Read the model definition and answer for the solid it produces. Units are mm, in the model's axes. Face numbers are marked on the shaded views. A direction names the side the tool comes from. Coordinates: 2 decimals unless noted, no trailing zeros. Loops run counter-clockwise (first coordinate to the right, second up) from the corner with the lowest first, then second, coordinate; pieces in that order, holes last. Notation, with made-up numbers: (62.25, 50) -> (110.25, 50) arc R13 ccw to (110.25, 74) -> close; hole circle Ø5 at (-17, 49). An arc over 180 degrees is marked (long way). Answer as CSV lines item,"result".
Autodesk Inventor part; units mm, degrees
ref_plane "YZ Plane" through (0, 0, 0) normal (1, 0, 0) x (0, 1, 0)
ref_plane "XZ Plane" through (0, 0, 0) normal (0, 1, 0) x (-1, 0, 0)
ref_plane "XY Plane" through (0, 0, 0) normal (0, 0, 1) x (1, 0, 0)
sketch "Arduino Uno" plane through (0, 0, 0) normal (0, 0, 1) x (1, 0, 0)
  line L0 (0, 0) -> (68.6, 0)
  line L1 (68.6, 0) -> (68.6, 53.3)
  line L2 (68.6, 53.3) -> (0, 53.3)
  line L3 (0, 53.3) -> (0, 0)
  circle A0 centre (14, 2.5) radius 1.6
  circle A1 centre (15.3, 50.7) radius 1.6
  circle A2 centre (66.1, 5.1) radius 1.6
  circle A3 centre (66.1, 33) radius 1.6
  dimension "d6" = 68.6
  dimension "d7" = 53.3
  dimension "d8" = 3.2
  dimension "d12" = 14
  dimension "d13" = 2.5
  dimension "d14" = 3.2
  dimension "d15" = 1.3
  dimension "d16" = 3.2
  dimension "d18" = 2.5
  dimension "d19" = 5.1
  dimension "d20" = 3.2
  dimension "d21" = 27.9
  dimension "d22" = 2.5
  dimension "d26" = 2.6
sketch "Sketch2" plane through (0, 0, 0) normal (0, 0, 1) x (1, 0, 0)
  line L0 (-7.6136, -10.2044) -> (-7.6136, 63.0956)
  line L1 (-7.6136, 63.0956) -> (106.3864, 63.0956)
  line L2 (106.3864, 63.0956) -> (106.3864, -10.2044)
  line L3 (106.3864, -10.2044) -> (-7.6136, -10.2044)
  dimension "d29" = 114
  dimension "d39" = 73.3
extrude "Back Plate" add sketch "Sketch2" against normal blind 10
extrude "Uno Mounting Holes" cut sketch "Arduino Uno" against normal blind 5 contours A0 | A1 | A2 | A3
sketch "3.5\" TFT LCD Screen" plane through (0, 0, 0) normal (0, 0, 1) x (1, 0, 0)
  line L0 (88.6005, 0.0003) -> (88.6005, 53.3003)
  line L1 (88.6005, 53.3003) -> (10.6005, 53.3003)
  line L2 (10.6005, 53.3003) -> (10.6005, 0.0003)
  line L3 (10.6005, 0.0003) -> (88.6005, 0.0003)
  circle A0 centre (66.1, 5.1) radius 1.6
  circle A1 centre (14, 2.5) radius 1.6
  circle A2 centre (15.3, 50.7) radius 1.6
  circle A3 centre (66.1, 33) radius 1.6
  line L4 (-7.6136, -10.2044) -> (-7.6136, 63.0956)
  line L5 (106.3864, -10.2044) -> (-7.6136, -10.2044)
  line L6 (106.3864, 63.0956) -> (106.3864, -10.2044)
  line L7 (-7.6136, 63.0956) -> (106.3864, 63.0956)
  point P0 (0, 0)
  point P1 (68.6, 0)
  dimension "d35" = 78
  dimension "d36" = 53.3
  dimension "d37" = 78
  dimension "d38" = 53.3
sketch "SD Card Slot" plane through (0, 0, 0) normal (0, 0, 1) x (1, 0, 0)
  line L0 (43.3864, 9.1) -> (-7.6136, 9.1)
  line L1 (-7.6136, 9.1) -> (-7.6136, 44.1)
  line L2 (-7.6136, 44.1) -> (43.3864, 44.1)
  line L3 (43.3864, 44.1) -> (43.3864, 9.1)
  circle A0 centre (14, 2.5) radius 1.6
  line L4 (-7.6136, -10.2044) -> (-7.6136, 63.0956)
  circle A1 centre (15.3, 50.7) radius 1.6
  point P0 (0, 0)
  dimension "d41" = 35
  dimension "d42" = 51
  dimension "d44" = 6.6
  dimension "d45" = 0
sketch "Sketch5" plane through (0, 0, 0) normal (0, 0, 1) x (1, 0, 0)
  line L0 (43.3864, 9.1) -> (-7.6136, 9.1)
  line L1 (43.3864, 44.1) -> (43.3864, 9.1)
  line L2 (-7.6136, 44.1) -> (43.3864, 44.1)
  line L3 (-7.6136, 9.1) -> (-7.6136, 44.1)
  line L4 (44.3864, 8.1) -> (44.3864, 45.1)
  line L5 (44.3864, 8.1) -> (-7.6136, 8.1)
  line L6 (-7.6136, -10.2044) -> (-7.6136, 63.0956)
  line L7 (44.3864, 45.1) -> (-7.6136, 45.1)
  line L8 (-7.6136, 45.1) -> (-7.6136, 47.6)
  line L9 (-7.6136, 47.6) -> (47.3864, 47.6)
  line L10 (-7.6136, 8.1) -> (-7.6136, 5.6)
  line L11 (-7.6136, 5.6) -> (47.3864, 5.6)
  line L12 (47.3864, 5.6) -> (47.3864, 47.6)
  point P0 (0, 0)
  dimension "d47" = 2.5
  dimension "d48" = 55
  dimension "d49" = 2.5
extrude "SD Card Slot Slot" add sketch "Sketch5" along normal blind 10 contours L5 L4 L7 L6 L9 L12 L11
sketch "Sketch6" plane through (47.3864, 5.6, 0) normal (1, 0, 0) x (0, 0, -1)
  line L0 (0, 42) -> (0, 0)
  line L1 (0, 42) -> (-10, 42)
  line L2 (-10, 0) -> (-10, 42)
  line L3 (0, 0) -> (-10, 0)
  line L4 (-6, 38) -> (-4, 38)
  line L5 (-4, 38) -> (-4, 4)
  line L6 (-4, 4) -> (-6, 4)
  line L7 (-6, 4) -> (-6, 38)
  point P0 (0, -5.6)
  dimension "d52" = 4
extrude "SD Ribbon Slot" cut sketch "Sketch6" against normal through all contours L4 L5 L6 L7
fillet "1.2mm Fillet" radius 1.2 7 edges at (19.8864, 47.6, 0) (19.8864, 5.6, 0) (47.3864, 26.6, 0) (47.3864, 5.6, 5) (47.3864, 47.6, 5) (44.3864, 45.1, 5) (44.3864, 8.1, 5)
sketch "Sketch7" plane through (0, 0, 0) normal (0, 0, 1) x (1, 0, 0)
  line L0 (106.3864, -10.2044) -> (101.3864, -10.2044)
  line L1 (101.3864, -10.2044) -> (101.3864, -5.2044)
  line L2 (101.3864, -5.2044) -> (106.3864, -5.2044)
  line L3 (106.3864, -5.2044) -> (106.3864, -10.2044)
  line L4 (49.3864, -10.2044) -> (49.3864, 80.0118)
  line L5 (-7.6136, 63.0956) -> (106.3864, 63.0956)
  line L6 (106.3864, 26.4456) -> (-34.6963, 26.4456)
  line L7 (-7.6136, -10.2044) -> (-2.6136, -10.2044)
  line L8 (-2.6136, -10.2044) -> (-2.6136, -5.2044)
  line L9 (-2.6136, -5.2044) -> (-7.6136, -5.2044)
  line L10 (-7.6136, -5.2044) -> (-7.6136, -10.2044)
  line L11 (106.3864, 63.0956) -> (101.3864, 63.0956)
  line L12 (101.3864, 63.0956) -> (101.3864, 58.0956)
  line L13 (101.3864, 58.0956) -> (106.3864, 58.0956)
  line L14 (106.3864, 58.0956) -> (106.3864, 63.0956)
  line L15 (-7.6136, 63.0956) -> (-2.6136, 63.0956)
  line L16 (-2.6136, 63.0956) -> (-2.6136, 58.0956)
  line L17 (-2.6136, 58.0956) -> (-7.6136, 58.0956)
  line L18 (-7.6136, 58.0956) -> (-7.6136, 63.0956)
  point P0 (0, 0)
  point P1 (0, 52.8913)
  dimension "d56" = 5
  dimension "d57" = 5
  dimension "d58" = 57
  dimension "d59" = 36.65
extrude "Pillars" add sketch "Sketch7" along normal blind 31
sketch "Sketch8" plane through (0, 0, 31) normal (0, 0, 1) x (1, 0, 0)
  line L0 (101.3864, -10.2044) -> (-2.6136, -10.2044)
  line L1 (-7.6136, -5.2044) -> (-2.6136, -5.2044)
  line L2 (101.3864, -10.2044) -> (-2.6136, -10.2044)
  line L3 (-2.6136, -10.2044) -> (-2.6136, -5.2044)
  line L4 (-2.6136, -5.2044) -> (101.3864, -5.2044)
  line L5 (101.3864, -5.2044) -> (101.3864, -10.2044)
  line L6 (101.3864, 63.0956) -> (101.3864, 58.0956)
  line L7 (106.3864, 63.0956) -> (106.3864, -10.2044)
  line L8 (101.3864, 58.0956) -> (106.3864, 58.0956)
  line L9 (106.3864, 58.0956) -> (106.3864, -5.2044)
  line L10 (106.3864, -5.2044) -> (101.3864, -5.2044)
  line L11 (101.3864, -5.2044) -> (101.3864, 58.0956)
  line L12 (-7.6136, 58.0956) -> (-2.6136, 58.0956)
  line L13 (-7.6136, 63.0956) -> (106.3864, 63.0956)
  line L14 (-2.6136, 58.0956) -> (101.3864, 58.0956)
  line L15 (101.3864, 58.0956) -> (101.3864, 63.0956)
  line L16 (101.3864, 63.0956) -> (-2.6136, 63.0956)
  line L17 (-2.6136, 63.0956) -> (-2.6136, 58.0956)
  line L18 (-2.6136, 58.0956) -> (-7.6136, 58.0956)
  line L19 (-7.6136, 58.0956) -> (-7.6136, -5.2044)
  line L20 (-7.6136, -5.2044) -> (-2.6136, -5.2044)
  line L21 (-2.6136, -5.2044) -> (-2.6136, 58.0956)
  point P0 (0, 0)
extrude "Beams (Will they print?)" [suppressed]
properties part number "Back Plate test03"
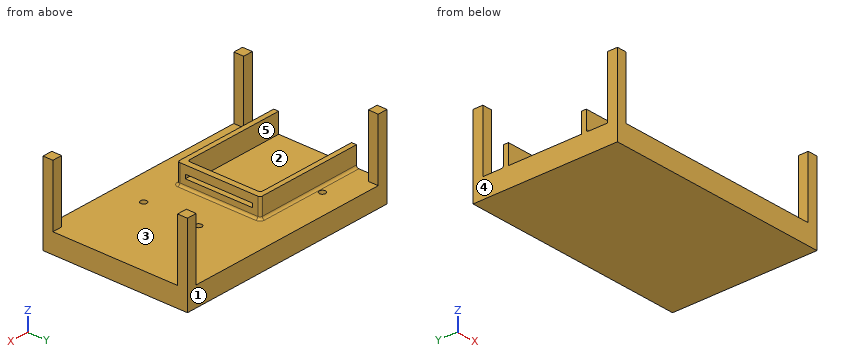
Q1. For the marked faces 1 and 2, determine the directions among +Z, -Z, +X, -X, +Y, -Y from which every point of the face is accessible in a straight line to the end or side of a thin tool.
Results:
face 1,"+Z, -Z, +X, -X, +Y"
face 2,"+Z, -X"
Q2. A cutting plane is placed at A-A, the plane y = 33. Write down the section's boundary in (x, z), and give its area (3 significant figures).
Results:
outline,"(-7.61, -10) -> (106.39, -10) -> (106.39, 0) -> (67.7, 0) -> (67.7, -5) -> (64.5, -5) -> (64.5, 0) -> (48.59, 0) arc R1.2 cw to (47.39, 1.2) -> (47.39, 4) -> (44.39, 4) -> (44.39, 0) -> (-7.61, 0) -> close; (44.39, 6) -> (47.39, 6) -> (47.39, 10) -> (44.39, 10) -> close"
area,"1,150 mm²"
Q3. For a pull along X with two mould halves and no side action, classify the marked faces 3, 4 and 5 as pulls with the +X half, pulls with the -X half, needs draft (parallel to the pull), parting line crosses it, or undercut.
Results:
face 3,"undercut"
face 4,"pulls with the -X half"
face 5,"needs draft"
Q4. A cutting plane is placed at D-D, the plane y = 24. Write down the section's boundary in (x, z), and give its area (3 significant figures).
Results:
outline,"(-7.61, -10) -> (106.39, -10) -> (106.39, 0) -> (48.59, 0) arc R1.2 cw to (47.39, 1.2) -> (47.39, 4) -> (44.39, 4) -> (44.39, 0) -> (-7.61, 0) -> close; (44.39, 6) -> (47.39, 6) -> (47.39, 10) -> (44.39, 10) -> close"
area,"1,160 mm²"
Q5. Given pin 1 Ø2 at (x, z) = (46.5, 5) entering from +Y; pin 2 Ø7 at (x, z) = (21, 4) entering from -Y; pin 3 Ø1 at (x, y) = (14.5, 51) entering from +Z, each flat-ended and moving along its own axis, determine where each tip first touches the part or whether it passes through.
Results:
pin 1,"stops at y = 47.6"
pin 2,"stops at y = 5.37"
pin 3,"stops at z = -5"
Q6. A cutting plane is placed at B-B, the plane z = 17. Write down the section's boundary in (x, y).
Results:
outline,"(-7.61, -10.2) -> (-2.61, -10.2) -> (-2.61, -5.2) -> (-7.61, -5.2) -> close; (-7.61, 58.1) -> (-2.61, 58.1) -> (-2.61, 63.1) -> (-7.61, 63.1) -> close; (101.39, -10.2) -> (106.39, -10.2) -> (106.39, -5.2) -> (101.39, -5.2) -> close; (101.39, 58.1) -> (106.39, 58.1) -> (106.39, 63.1) -> (101.39, 63.1) -> close"
Q7. Find the intervals of material crossed by probe 1 along Y at (x, z) = (66.1, -3.55); probe 2 along Z at (x, y) = (71.5, 24.5); probe 3 along Y at (x, z) = (4.5, 8.5), in increasing order. Write a range as [from, to].
Results:
probe 1,"y = [-10.2, 3.5], [6.7, 31.4], [34.6, 63.1]"
probe 2,"z = [-10, 0]"
probe 3,"y = [5.6, 8.1], [45.1, 47.6]"
Q8. A cutting plane is placed at C-C, the plane y = 50.7. Write down the section's boundary in (x, z), and give its area (3 significant figures).
Results:
outline,"(-7.61, -10) -> (106.39, -10) -> (106.39, 0) -> (16.9, 0) -> (16.9, -5) -> (13.7, -5) -> (13.7, 0) -> (-7.61, 0) -> close"
area,"1,120 mm²"
